Input: part model. Units: mm. Frame: model coordinates. A direction names the side the tool comes from. Round coordinates to 2 decimals unless told otherwise and drop trailing zeros. Order: outer loops, then holes, each group sorted by start corner. A loop starts at its lowest first (then second) coordinate and runs counter-clockwise, first axis right, second up. Notation, with made-up numbers: (54.25, -8) -> (106.25, -8) arc R9 cw to (106.25, 9) -> close; hole circle Ø3 at (86, 82). An arc over 180 degrees is marked (long way). Use a Markdown table: item, result.
from build123d import *

# Parameters (mm, degrees)
SALIENTE_EXTRUIR1_DEPTH                = 10
CROQUIS5_W                             = 37
CROQUIS5_H                             = 22.5
CORTAR_EXTRUIR1_DEPTH                  = 5
TALADRO_DE_MARGEN_PARA_M31_D           = 3.4
TALADRO_DE_MARGEN_PARA_M31_CSINK_D     = 3.45
TALADRO_DE_MARGEN_PARA_M31_CSINK_ANGLE = 90
SALIENTE_EXTRUIR2_DEPTH                = 62
SALIENTE_EXTRUIR3_DEPTH                = 10
REDONDEO2_R                            = 10
CORTAR_EXTRUIR2_DEPTH                  = 10
CORTAR_EXTRUIR3_START                  = -10
CORTAR_EXTRUIR3_DEPTH                  = 10
TALADRO_DE_MARGEN_PARA_M61_D           = 6.6
TALADRO_DE_MARGEN_PARA_M61_CSINK_D     = 6.65
TALADRO_DE_MARGEN_PARA_M61_CSINK_ANGLE = 90
TALADRO_START                          = -130.385063418
TALADRO_DE_MARGEN_PARA_M62_OUTLINE_R   = 3.3
TALADRO_DE_MARGEN_PARA_M62_DEPTH       = 10.491681749
CROQUIS25_R                            = 12.5
SALIENTE_EXTRUIR4_DEPTH                = 10
SALIENTE_EXTRUIR5_START                = -10
CROQUIS26_R                            = 12.5
SALIENTE_EXTRUIR5_DEPTH                = 10
TALADRO_DE_MARGEN_PARA_M51_D           = 5.5
SALIENTE_EXTRUIR6_DEPTH                = 10
REDONDEO3_R                            = 2


# Read off the part's stored shape, not the designer's step: Taladro de margen para M62
with BuildPart() as part:
    # Croquis1 → Saliente-Extruir1 (new body)
    with BuildSketch(Plane(origin=(0, 0, 0), x_dir=(1, 0, 0), z_dir=(0, 1, 0))):
        with BuildLine():
            Line((-97.75, 169.30796644), (-60.25, 104.356061156))
            ThreePointArc((-60.25, 104.356061156), (0, 120.5), (60.25, 104.356061156))
            Line((60.25, 104.356061156), (97.75, 169.30796644))
            ThreePointArc((97.75, 169.30796644), (0, 195.5), (-97.75, 169.30796644))
        make_face()
    extrude(amount=SALIENTE_EXTRUIR1_DEPTH)

    # Croquis5 → Cortar-Extruir1 (cut)
    with BuildSketch(Plane.XZ):
        with Locations((0, -158)):
            Rectangle(CROQUIS5_W, CROQUIS5_H)
    extrude(amount=-CORTAR_EXTRUIR1_DEPTH, mode=Mode.SUBTRACT)

    # Taladro de margen para M31 (through all)
    with Locations(Plane(origin=(0, 5, 0), x_dir=(-1, 0, 0), z_dir=(0, -1, 0))):
        with Locations((-15, 165.5), (-15, 150.5), (15, 150.5), (15, 165.5)):
            CounterSinkHole(TALADRO_DE_MARGEN_PARA_M31_D / 2, TALADRO_DE_MARGEN_PARA_M31_CSINK_D / 2, counter_sink_angle=TALADRO_DE_MARGEN_PARA_M31_CSINK_ANGLE)

    # Croquis14 → Saliente-Extruir2 (add)
    with BuildSketch(Plane(origin=(0, 10, 0), x_dir=(1, 0, 0), z_dir=(0, 1, 0))):
        with BuildLine():
            Line((-65.25, 113.016315194), (-60.25, 104.356061156))
            ThreePointArc((-60.25, 104.356061156), (0, 120.5), (60.25, 104.356061156))
            Line((60.25, 104.356061156), (65.25, 113.016315194))
            ThreePointArc((65.25, 113.016315194), (0, 130.5), (-65.25, 113.016315194))
        make_face()
    extrude(amount=SALIENTE_EXTRUIR2_DEPTH)

    # Croquis15 → Saliente-Extruir3 (add)
    with BuildSketch(Plane(origin=(0, 72, 0), x_dir=(1, 0, 0), z_dir=(0, 1, 0))):
        with BuildLine():
            Line((-97.75, 169.30796644), (-60.25, 104.356061156))
            ThreePointArc((-60.25, 104.356061156), (0, 120.5), (60.25, 104.356061156))
            Line((60.25, 104.356061156), (97.75, 169.30796644))
            ThreePointArc((97.75, 169.30796644), (0, 195.5), (-97.75, 169.30796644))
        make_face()
    extrude(amount=SALIENTE_EXTRUIR3_DEPTH)

    # Redondeo2
    redondeo2_edges = [part.edges().sort_by_distance(p)[0] for p in [
        (0, 10, -130.5),
        (0, 72, -130.5),
    ]]
    fillet(redondeo2_edges, radius=REDONDEO2_R)

    # Croquis16 → Cortar-Extruir2 (cut)
    with BuildSketch(Plane(origin=(0, 82, 0), x_dir=(1, 0, 0), z_dir=(0, 1, 0))):
        with BuildLine():
            Line((-78.395687553, 168.120094495), (-72.056413627, 154.52547769))
            ThreePointArc((-72.056413627, 154.52547769), (-54.805428834, 161.451587079), (-36.902954176, 166.458469214))
            Line((-36.902954176, 166.458469214), (-40.149548386, 181.102909321))
            ThreePointArc((-40.149548386, 181.102909321), (-59.627020814, 175.655539021), (-78.395687553, 168.120094495))
        make_face()
        with BuildLine():
            Line((-65.717139701, 140.930860884), (-59.377865775, 127.336244079))
            ThreePointArc((-59.377865775, 127.336244079), (-45.162244875, 133.043683194), (-30.409765758, 137.169589))
            Line((-30.409765758, 137.169589), (-33.656359967, 151.814029107))
            ThreePointArc((-33.656359967, 151.814029107), (-49.983836855, 147.247635136), (-65.717139701, 140.930860884))
        make_face()
        with BuildLine():
            Line((-24.212608657, 183.913021785), (-22.254715774, 169.041348864))
            ThreePointArc((-22.254715774, 169.041348864), (0, 170.5), (22.254715774, 169.041348864))
            Line((22.254715774, 169.041348864), (24.212608657, 183.913021785))
            ThreePointArc((24.212608657, 183.913021785), (0, 185.5), (-24.212608657, 183.913021785))
        make_face()
        with BuildLine():
            Line((-20.29682289, 154.169675944), (-18.338930007, 139.298003023))
            ThreePointArc((-18.338930007, 139.298003023), (0, 140.5), (18.338930007, 139.298003023))
            Line((18.338930007, 139.298003023), (20.29682289, 154.169675944))
            ThreePointArc((20.29682289, 154.169675944), (0, 155.5), (-20.29682289, 154.169675944))
        make_face()
        with BuildLine():
            Line((40.149548386, 181.102909321), (36.902954176, 166.458469214))
            ThreePointArc((36.902954176, 166.458469214), (54.805428834, 161.451587079), (72.056413627, 154.52547769))
            Line((72.056413627, 154.52547769), (78.395687553, 168.120094495))
            ThreePointArc((78.395687553, 168.120094495), (59.627020814, 175.655539021), (40.149548386, 181.102909321))
        make_face()
        with BuildLine():
            Line((33.656359967, 151.814029107), (30.409765758, 137.169589))
            ThreePointArc((30.409765758, 137.169589), (45.162244875, 133.043683194), (59.377865775, 127.336244079))
            Line((59.377865775, 127.336244079), (65.717139701, 140.930860884))
            ThreePointArc((65.717139701, 140.930860884), (49.983836855, 147.247635136), (33.656359967, 151.814029107))
        make_face()
    extrude(amount=-CORTAR_EXTRUIR2_DEPTH, mode=Mode.SUBTRACT)

    # Croquis19 → Cortar-Extruir3 (cut)
    with BuildSketch(Plane.XZ.offset(CORTAR_EXTRUIR3_START)):
        with BuildLine():
            Line((72.056413627, -154.52547769), (78.395687553, -168.120094495))
            ThreePointArc((78.395687553, -168.120094495), (59.627020814, -175.655539021), (40.149548386, -181.102909321))
            Line((40.149548386, -181.102909321), (36.902954176, -166.458469214))
            ThreePointArc((36.902954176, -166.458469214), (54.805428834, -161.451587079), (72.056413627, -154.52547769))
        make_face()
        with BuildLine():
            Line((59.377865775, -127.336244079), (65.717139701, -140.930860884))
            ThreePointArc((65.717139701, -140.930860884), (49.983836855, -147.247635136), (33.656359967, -151.814029107))
            Line((33.656359967, -151.814029107), (30.409765758, -137.169589))
            ThreePointArc((30.409765758, -137.169589), (45.162244875, -133.043683194), (59.377865775, -127.336244079))
        make_face()
        with BuildLine():
            Line((-78.395687553, -168.120094495), (-72.056413627, -154.52547769))
            ThreePointArc((-72.056413627, -154.52547769), (-54.805428834, -161.451587079), (-36.902954176, -166.458469214))
            Line((-36.902954176, -166.458469214), (-40.149548386, -181.102909321))
            ThreePointArc((-40.149548386, -181.102909321), (-59.627020814, -175.655539021), (-78.395687553, -168.120094495))
        make_face()
        with BuildLine():
            Line((-65.717139701, -140.930860884), (-59.377865775, -127.336244079))
            ThreePointArc((-59.377865775, -127.336244079), (-45.162244875, -133.043683194), (-30.409765758, -137.169589))
            Line((-30.409765758, -137.169589), (-33.656359967, -151.814029107))
            ThreePointArc((-33.656359967, -151.814029107), (-49.983836855, -147.247635136), (-65.717139701, -140.930860884))
        make_face()
    extrude(amount=CORTAR_EXTRUIR3_DEPTH, mode=Mode.SUBTRACT)

    # Taladro de margen para M61 (through all)
    with Locations(Plane(origin=(33.775885386, 0, -126.053320331), x_dir=(0, -1, 0), z_dir=(0.2588190451025245, 0, -0.9659258262890673))):
        with Locations((-57, -8.775885386)):
            CounterSinkHole(TALADRO_DE_MARGEN_PARA_M61_D / 2, TALADRO_DE_MARGEN_PARA_M61_CSINK_D / 2, counter_sink_angle=TALADRO_DE_MARGEN_PARA_M61_CSINK_ANGLE)

    # Taladro de margen para M62 outline → Taladro de margen para M62 (cut)
    with BuildSketch(Plane(origin=(0, 0, 0), x_dir=(0.9659258262890672, 0, -0.2588190451025251), z_dir=(0.25881904510252507, 0, 0.9659258262890672)).offset(TALADRO_START)):
        with Locations((-8.775885386, 25)):
            Circle(TALADRO_DE_MARGEN_PARA_M62_OUTLINE_R)
    extrude(amount=TALADRO_DE_MARGEN_PARA_M62_DEPTH, mode=Mode.SUBTRACT)

    # Croquis25 → Saliente-Extruir4 (add)
    with BuildSketch(Plane(origin=(0, 82, 0), x_dir=(1, 0, 0), z_dir=(0, 1, 0))):
        with Locations((-52.394632844, 154.349611108)):
            Circle(CROQUIS25_R)
        with Locations((52.394632844, 154.349611108)):
            Circle(CROQUIS25_R)
    extrude(amount=-SALIENTE_EXTRUIR4_DEPTH)

    # Croquis26 → Saliente-Extruir5 (add)
    with BuildSketch(Plane.XZ.offset(SALIENTE_EXTRUIR5_START)):
        with Locations((-52.394632844, -154.349611108)):
            Circle(CROQUIS26_R)
        with Locations((52.394632844, -154.349611108)):
            Circle(CROQUIS26_R)
    extrude(amount=SALIENTE_EXTRUIR5_DEPTH)

    # Taladro de margen para M51 (through all)
    with Locations(Plane(origin=(0, 82, 0), x_dir=(1, 0, 0), z_dir=(0, 1, 0))):
        with Locations((-52.394632844, 154.349611108), (52.394632844, 154.349611108)):
            Hole(TALADRO_DE_MARGEN_PARA_M51_D / 2)

    # Croquis29 → Saliente-Extruir6 (add)
    with BuildSketch(Plane(origin=(0, 82, 0), x_dir=(1, 0, 0), z_dir=(0, 1, 0))):
        with BuildLine():
            Line((-82.926991651, 191.845896293), (-79.618434834, 190.55905839))
            ThreePointArc((-79.618434834, 190.55905839), (-71.00972345, 182.317098184), (-71.269055695, 194.232322333))
            Line((-71.269055695, 194.232322333), (-69.982217792, 197.54087915))
            ThreePointArc((-69.982217792, 197.54087915), (-69.580152297, 179.067663415), (-82.926991651, 191.845896293))
        make_face()
    extrude(amount=-SALIENTE_EXTRUIR6_DEPTH)

    # Redondeo3
    # the kernel refuses this fillet: 2 mm, written as the material it takes off along each edge
    with BuildSketch(Plane(origin=(-69.982217792, 88.300214624, -197.54087915), x_dir=(0.8788843703548711, 0, 0.477034866174289), z_dir=(0, -1, 0))) as redondeo3_piece_1:
        with BuildLine():
            CenterArc((2.268077265, 1.984059393), REDONDEO3_R, 172.761243907, 104.477512186)
            Line((0.284017872, 2.236067977), (0, 0))
            ThreePointArc((0, 0), (1.260042925, -0.079703037), (2.52008585, 0))
        make_face()
    extrude(amount=22.600429248, mode=Mode.SUBTRACT)
    with BuildSketch(Plane(origin=(-71.269055695, 86.399756393, -194.232322333), x_dir=(0.3624895501390437, 0, -0.9319878357789836), z_dir=(0, -1, 0))) as redondeo3_piece_2:
        with BuildLine():
            CenterArc((1.759902557, 2), REDONDEO3_R, 193.691050596, 76.308949404)
            ThreePointArc((-0.183269646, 1.526627219), (-0.045981309, 0.768794255), (0, 0))
            Line((0, 0), (1.759902557, 0))
        make_face()
    extrude(amount=18.799512786, mode=Mode.SUBTRACT)
    with BuildSketch(Plane(origin=(-79.618434834, 86.399756393, -190.55905839), x_dir=(-0.931987835778983, 0, -0.3624895501390453), z_dir=(0, -1, 0))) as redondeo3_piece_3:
        with BuildLine():
            CenterArc((1.759902557, -2), REDONDEO3_R, 90, 76.308949404)
            ThreePointArc((-0.183269646, -1.526627219), (-0.045981309, -0.768794255), (0, 0))
            Line((0, 0), (1.759902557, 0))
        make_face()
    extrude(amount=18.799512786, mode=Mode.SUBTRACT)
    with BuildSketch(Plane(origin=(-82.926991651, 88.300214624, -191.845896293), x_dir=(-0.2421659304746274, 0, 0.9702348489501693), z_dir=(0, -1, 0))) as redondeo3_piece_4:
        with BuildLine():
            CenterArc((2.268077265, -1.984059393), REDONDEO3_R, 82.761243907, 104.477512186)
            Line((0.284017872, -2.236067977), (0, 0))
            ThreePointArc((0, 0), (1.260042925, 0.079703037), (2.52008585, 0))
        make_face()
    extrude(amount=22.600429248, mode=Mode.SUBTRACT)


solid = part.part
1) Ray query, probe 1 along Z at (x, y) = (-1, 74.5); probe 2 along Y at (x, z) = (29, -183.5); probe 3 along Z at (x, y) = (-15, 8.8). Return the intervals inside material, ascending.
Answer key:
| item | result |
|---|---|
| probe 1 | z = -195.5 to -185.5, -170.5 to -155.5, -140.5 to -120.5 |
| probe 2 | y = 0 to 10, 72 to 82 |
| probe 3 | z = -194.92 to -167.2, -163.8 to -152.2, -148.8 to -119.56 |
2) Draft query along X for faces 1 (the face through (-37.11, 77.07, -151.007)), 2 (the face through (-1, 10, -159)). Return one class per face: released by +X, released by -X, zero draft, split by the parting line, or undercut.
Answer key:
| item | result |
|---|---|
| face 1 | undercut |
| face 2 | zero draft |
3) Cut plane A-A on z = -172.5. Return loops of the section in (x, y).
Answer key:
| item | result |
|---|---|
| outline | (-92, 0) -> (-68.22, 0) -> (-68.22, 10) -> (-92, 10) -> close; (-92, 72) -> (-68.22, 72) -> (-68.22, 82) -> (-92, 82) -> close; (-38.24, 0) -> (38.24, 0) -> (38.24, 10) -> (-38.24, 10) -> close; (-38.24, 72) -> (-22.71, 72) -> (-22.71, 82) -> (-38.24, 82) -> close; (22.71, 72) -> (38.24, 72) -> (38.24, 82) -> (22.71, 82) -> close; (68.22, 0) -> (92, 0) -> (92, 10) -> (68.22, 10) -> close; (68.22, 72) -> (92, 72) -> (92, 82) -> (68.22, 82) -> close |
4) Cut plane B-B on x = 81.5. Return loops of the section in (y, z), and give its area (3 significant figures).
Answer key:
| item | result |
|---|---|
| outline | (0, -177.7) -> (10, -177.7) -> (10, -141.16) -> (0, -141.16) -> close; (72, -177.7) -> (82, -177.7) -> (82, -141.16) -> (72, -141.16) -> close |
| area | 731 mm^2 |
5) Contact query for flat-ended pins moving along their axis: P1, Ø4, axis at y = 3, z = -162, coming from the -X side; P2, Ø1, axis at x = 27, y = 37.5, coming from the -Z side; P3, Ø1.5, axis at x = 13.5, y = 40, coming from the -Z side; P4, Ø7, axis at x = 52.39, z = -154.35, coming from the -Y side. Output: stop coordinate, or through.
Answer key:
| item | result |
|---|---|
| P1 | stops at x = -94.69 |
| P2 | stops at z = -127.78 |
| P3 | stops at z = -129.88 |
| P4 | stops at y = 0 |
6) Cut plane C-C on y = 43. Return loops of the section in (x, z), and give its area (3 significant figures).
Answer key:
| item | result |
|---|---|
| outline | (-65.25, -113.02) arc R130.5 ccw to (65.25, -113.02) -> (60.25, -104.36) arc R120.5 cw to (-60.25, -104.36) -> close |
| area | 1,310 mm^2 |
7) Set-up query: faces 3 (the face through (0.3, 77.1, -185.5)), 4 (the face through (-18.5, 2, -158)), 5 (the face through (48.53, 5.07, -142.46)), 6 (the face through (-0.883, 40.426, -120.497)). Return all of +Z, -Z, +X, -X, +Y, -Y with unobstructed straight access to the full face (end or side cutting, diameter ignored); none if empty.
Answer key:
| item | result |
|---|---|
| face 3 | +Y |
| face 4 | -Y |
| face 5 | +Y, -Y |
| face 6 | +Z, +Y, -Y |
